```python
from build123d import *

# Parameters (mm, degrees)
SKETCH_1_R          = 33
EXTRUDE_1_DEPTH     = 2.5
SKETCH_2_R          = 30.35
EXTRUDE_2_DEPTH     = 11.5
SKETCH_3_R          = 33
EXTRUDE_3_DEPTH     = 2.5
SKETCH_4_R          = 24
EXTRUDE_4_DEPTH     = 9.5
CHAMFER_1_SIZE      = 1
SKETCH_5_R          = 5
CUT_EXTRUDE_1_DEPTH = 54.422841557
SKETCH_6_W          = 50
SKETCH_6_H          = 1.4
CUT_EXTRUDE_2_DEPTH = 9
SKETCH_7_R          = 2.75
CUT_EXTRUDE_3_DEPTH = 8
SKETCH_8_R          = 5
CUT_EXTRUDE_4_DEPTH = 60.193665202
HOLE_WIZARD_M5_1_D  = 4.2
SKETCH_12_W         = 10
SKETCH_12_H         = 14
CUT_EXTRUDE_5_DEPTH = 4
SKETCH_13_W         = 72.487869612
SKETCH_13_H         = 16.576438216
CUT_EXTRUDE_6_DEPTH = 9.3


with BuildPart() as part:
    # 草图1 → 凸台-拉伸1 (new body)
    with BuildSketch(Plane.XY):
        Circle(SKETCH_1_R)
    extrude(amount=EXTRUDE_1_DEPTH)

    # 草图2 → 凸台-拉伸2 (add)
    with BuildSketch(Plane.XY.offset(2.5)):
        Circle(SKETCH_2_R)
    extrude(amount=EXTRUDE_2_DEPTH)

    # 草图3 → 凸台-拉伸3 (add)
    with BuildSketch(Plane.XY.offset(14)):
        Circle(SKETCH_3_R)
    extrude(amount=EXTRUDE_3_DEPTH)

    # 草图4 → 凸台-拉伸4 (add)
    with BuildSketch(Plane.XY.offset(16.5)):
        Circle(SKETCH_4_R)
    extrude(amount=EXTRUDE_4_DEPTH)

    # 倒角1
    chamfer_1_edges = [part.edges().sort_by_distance(p)[0] for p in [
        (-33, 0, 2.5),
        (-33, 0, 14),
    ]]
    chamfer(chamfer_1_edges, length=CHAMFER_1_SIZE)

    # 草图5 → 切除-拉伸1 (cut, through all)
    with BuildSketch(Plane.XY.offset(26)):
        Circle(SKETCH_5_R)
    extrude(amount=-CUT_EXTRUDE_1_DEPTH, mode=Mode.SUBTRACT)

    # 草图6 → 切除-拉伸2 (cut)
    with BuildSketch(Plane.XY.offset(26)):
        Rectangle(SKETCH_6_W, SKETCH_6_H)
    extrude(amount=-CUT_EXTRUDE_2_DEPTH, mode=Mode.SUBTRACT)

    # 草图7 → 切除-拉伸3 (cut)
    with BuildSketch(Plane.XZ.offset(-0.7)):
        with Locations((-13, 22)):
            Circle(SKETCH_7_R)
        with Locations(Location((13, 22, 0), (0, 0, 180))):
            Circle(SKETCH_7_R)
    extrude(amount=-CUT_EXTRUDE_3_DEPTH, mode=Mode.SUBTRACT)

    # 草图8 → 切除-拉伸4 (cut, through all)
    with BuildSketch(Plane.XZ.offset(-8.7)):
        with Locations((-13, 22)):
            Circle(SKETCH_8_R)
        with Locations((13, 22)):
            Circle(SKETCH_8_R)
    extrude(amount=-CUT_EXTRUDE_4_DEPTH, mode=Mode.SUBTRACT)

    # M5 螺纹孔1 (through all)
    with Locations(Plane(origin=(0, -0.7, 0), x_dir=(-1, 0, 0), z_dir=(0, 1, 0))):
        with Locations((13, 22), (-13, 22)):
            Hole(HOLE_WIZARD_M5_1_D / 2)

    # 草图12 → 切除-拉伸5 (cut)
    with BuildSketch(Plane.XY.offset(26)):
        with Locations((-13, 15.7)):
            Rectangle(SKETCH_12_W, SKETCH_12_H)
        with Locations((13, 15.7)):
            Rectangle(SKETCH_12_W, SKETCH_12_H)
    extrude(amount=-CUT_EXTRUDE_5_DEPTH, mode=Mode.SUBTRACT)

    # 草图13 → 切除-拉伸6 (cut)
    with BuildSketch(Plane.XY.offset(26)):
        with Locations((-2.709766805, 16.988219108)):
            Rectangle(SKETCH_13_W, SKETCH_13_H)
    extrude(amount=-CUT_EXTRUDE_6_DEPTH, mode=Mode.SUBTRACT)


solid = part.part
```
Could you check a few things on this model? Use its own coordinates, in mm. A direction names the side the tool comes from. Round coordinates to 2 decimals unless told otherwise and drop trailing zeros. Loops run counter-clockwise (first coordinate to the right, second up) from the corner with the lowest first, then second, coordinate; pieces in that order, holes last.
Q1. Please list where these lines run through material, in increasing order: L1, parallel to Z at x = 13, y = 3; L2, parallel to Z at x = 13, y = -8.5; L3, parallel to Z at x = -26, y = 5.
Q2. I want a section at C-C (z = 6.5). Write out the boundary of the cut face in (x, y).
Q3. For P1, Ø2, axis at y = -14, z = 12, coming from the -X side; P2, Ø0.7, axis at x = -14, y = 0, coming from the +Z side; P3, Ø7, axis at x = -13, z = 22, coming from the -Y side; P4, Ø4, axis at x = -13, z = 22, coming from the -Y side, each with a flat end and sliding along its axis, tell me the tip position at first contact or that it passes through.
Q4. I want a section at A-A (x = 0). Write out the boundary of the cut face in (y, z).
Q5. I want a section at B-B (z = 22). Write out the boundary of the cut face in (x, y), and give its area (3 significant figures).
Q6. Thinking about a two-plate mould opening in Y: for faces 6 (the cylindrical face through (-5.2, -23.43, 21.18)), 7 (the flat face through (0, -7, 0)), 8 (the flat face through (-17, 0.7, 22)), 9 (the flat face through (-15, -0.7, 20)), which applies, pulls with the +Y half, pulls with the -Y half, needs draft (parallel to the pull), parting line crosses it, or undercut?
Q7. I want a section at D-D (y = 6). Give the number of separate pieces and of enclosed holes in the cut face, and give its area (3 significant figures).
Q8. On a 3-axis mill with a long thin cutter (end or side, diameter ignored), from which of +Z, -Z, +X, -X, +Y, -Y can I reach the whole of each face in a straight line? I mean faces 1 (the cylindrical face through (28.948, 9.116, 8.169)), 2 (the flat face through (16, 0.7, 22)), 3 (the flat face through (0, 8.7, 21)), 4 (the flat face through (2.3, -24.3, 16.5)), 5 (the cylindrical face through (13.358, 4.644, 19.273)). Say none if no direction works.
Answer below:
1. L1: z = 0 to 19.25, 24.75 to 26
1. L2: z = 0 to 19.9, 24.1 to 26
1. L3: z = 0 to 16.5
2. outline: circle Ø60.7 at (0, 0); hole circle Ø10 at (0, 0)
3. P1: stops at x = -27.42
3. P2: stops at z = 17
3. P3: stops at y = -22.04
3. P4: passes through
4. outline: (-33, 0) - (-5, 0) - (-5, 26) - (-24, 26) - (-24, 16.5) - (-33, 16.5) - (-33, 15) - (-32, 14) - (-30.35, 14) - (-30.35, 2.5) - (-32, 2.5) - (-33, 1.5) - close; (5, 0) - (33, 0) - (33, 1.5) - (32, 2.5) - (30.35, 2.5) - (30.35, 14) - (32, 14) - (33, 15) - (33, 16.5) - (24, 16.5) - (24, 16.7) - (8.7, 16.7) - (8.7, 26) - (5, 26) - close
5. outline: (-23.99, -0.7) arc R24 ccw to (-15.1, -18.65) - (-15.1, -0.7) - close; (-23.99, 0.7) - (-15.75, 0.7) - (-15.75, 8.7) - (-22.37, 8.7) arc R24 ccw to start; (-10.9, -21.38) arc R24 ccw to (10.9, -21.38) - (10.9, -0.7) - (4.95, -0.7) arc R5 cw to (-4.95, -0.7) - (-10.9, -0.7) - close; (-10.25, 0.7) - (-4.95, 0.7) arc R5 cw to (4.95, 0.7) - (10.25, 0.7) - (10.25, 8.7) - (-10.25, 8.7) - close; (15.1, -18.65) arc R24 ccw to (23.99, -0.7) - (15.1, -0.7) - close; (15.75, 0.7) - (23.99, 0.7) arc R24 ccw to (22.37, 8.7) - (15.75, 8.7) - close
5. area: 930 mm2
6. face 6: parting line crosses it
6. face 7: needs draft
6. face 8: undercut
6. face 9: undercut
7. separate pieces: 1
7. enclosed holes: 2
7. area: 1,400 mm2
8. face 1: none
8. face 2: +Z, +X, -X
8. face 3: +Z, +X, -X, +Y
8. face 4: +Z
8. face 5: +Y
